For this review, take the finished solid that the model builds, in its own axes (mm). Face numbers are marked on the shaded views. Coordinates: 2 decimals unless noted, no trailing zeros. Write each loop counter-clockwise with the first axis right and the second up, starting at its lowest first coordinate (ties: lowest second). Pieces come first, ordered by that corner, then holes. Notation, with made-up numbers: (34, 74.5) -> (65, 74.5) arc R20 cw to (65, 83.5) -> close; hole circle Ø2 at (20, -35). An arc over 180 degrees is marked (long way). One line per item, written item: value. Start each with the question number.
1) For pin 1 Ø1.5 at (x, z) = (-16, 3.5) entering from +Y; pin 2 Ø5 at (x, y) = (-8, -8.5) entering from -Z; pin 3 Ø3 at (x, y) = (-5.5, -2.5) entering from +Z; pin 4 Ø1.5 at (x, z) = (-18, 2) entering from -Y, all flat-tipped, find the tip position at first contact; note any pin that passes through.
2) Add section C-C (y = 9). State the section outline as (x, z) points.
3) Mouldability with a two-part tool opening along X and no side actions: class the marked faces 1, 2, 3 and 4 as released by +X, released by -X, zero draft, split by the parting line, or undercut.
4) For probe 1 along Y at (x, z) = (-12.5, 4.7); probe 2 along Z at (x, y) = (-5.5, -6); probe 3 along Y at (x, z) = (-5, 0.6) (3 decimals), list the stretches that pass through material, from the lowest coordinate up. Write a range as from..to.
5) Add section A-A (x = -3.75). State the section outline as (y, z) points, and give its area (3 significant figures).
6) Add section B-B (y = 0). State the section outline as (x, z) points, and give its area (3 significant figures).
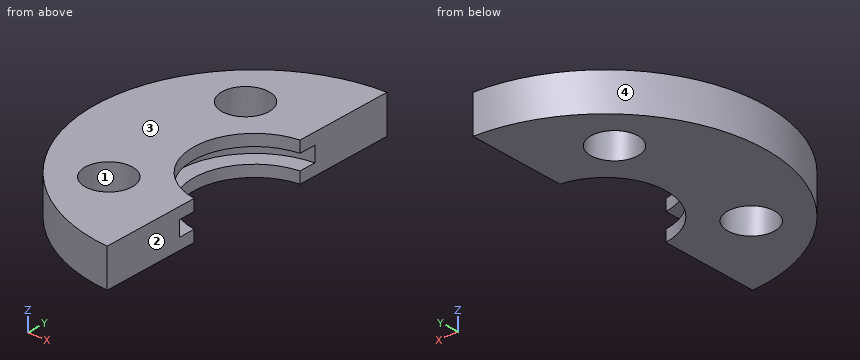
from build123d import *

# Parameters (mm, degrees)
SKETCH_1_R          = 21
SKETCH_1_R_2        = 3.1
SKETCH_1_R_3        = 8
EXTRUDE_1_DEPTH     = 5
CUT_EXTRUDE_1_DEPTH = 10
SKETCH_3_W          = 2
SKETCH_3_H          = 1.455022594
CUT_EXTRUDE_2_DEPTH = 2
SKETCH_4_R          = 10.2
CUT_EXTRUDE_3_DEPTH = 2


with BuildPart() as part:
    # 草图1 → 凸台-拉伸1 (new body)
    with BuildSketch(Plane.XY):
        Circle(SKETCH_1_R)
        with Locations((-10.253048327, 10.253048327)):
            Circle(SKETCH_1_R_2, mode=Mode.SUBTRACT)
        with Locations((10.253048327, 10.253048327)):
            Circle(SKETCH_1_R_2, mode=Mode.SUBTRACT)
        with Locations((-10.253048327, -10.253048327)):
            Circle(SKETCH_1_R_2, mode=Mode.SUBTRACT)
        with Locations((10.253048327, -10.253048327)):
            Circle(SKETCH_1_R_2, mode=Mode.SUBTRACT)
        Circle(SKETCH_1_R_3, mode=Mode.SUBTRACT)
    extrude(amount=EXTRUDE_1_DEPTH)

    # 草图2 → 切除-拉伸1 (cut)
    with BuildSketch(Plane.XY.offset(5)):
        Polygon((-1, 0), (-1, 23.542037427), (27.759132826, 23.542037427), (27.759132826, -27.308763415), (-1, -27.308763415), align=None)
    extrude(amount=-CUT_EXTRUDE_1_DEPTH, mode=Mode.SUBTRACT)

    # 草图3 → 切除-拉伸2 (cut)
    with BuildSketch(Plane(origin=(-1, 0, 0), x_dir=(0, 0, -1), z_dir=(1, 0, 0))):
        with Locations((-2.5, 7.937253933)):
            Rectangle(SKETCH_3_W, SKETCH_3_H)
    extrude(amount=-CUT_EXTRUDE_2_DEPTH, mode=Mode.SUBTRACT)

    # 草图4 → 切除-拉伸3 (cut)
    with BuildSketch(Plane.XY.offset(1.5)):
        Circle(SKETCH_4_R)
    extrude(amount=CUT_EXTRUDE_3_DEPTH, mode=Mode.SUBTRACT)


solid = part.part
Numbers:
1. pin 1: y = 14.44
1. pin 2: z = 0
1. pin 3: through
1. pin 4: y = -11.98
2. outline: (-18.97, 0) -> (-13.09, 0) -> (-13.09, 5) -> (-18.97, 5) -> close; (-7.42, 0) -> (-1, 0) -> (-1, 1.5) -> (-4.8, 1.5) -> (-4.8, 3.5) -> (-1, 3.5) -> (-1, 5) -> (-7.42, 5) -> close
3. face 1: undercut
3. face 2: released by +X
3. face 3: zero draft
3. face 4: released by -X
4. probe 1: -16.87..-12.39, -8.12..8.12, 12.39..16.87
4. probe 2: 0..1.5, 3.5..5
4. probe 3: -20.396..-6.245, 6.245..20.396
5. outline: (-20.66, 0) -> (-7.07, 0) -> (-7.07, 1.5) -> (-9.49, 1.5) -> (-9.49, 3.5) -> (-7.07, 3.5) -> (-7.07, 5) -> (-20.66, 5) -> close; (7.07, 0) -> (20.66, 0) -> (20.66, 5) -> (7.07, 5) -> (7.07, 3.5) -> (9.49, 3.5) -> (9.49, 1.5) -> (7.07, 1.5) -> close
5. area: 126 mm²
6. outline: (-21, 0) -> (-8, 0) -> (-8, 1.5) -> (-10.2, 1.5) -> (-10.2, 3.5) -> (-8, 3.5) -> (-8, 5) -> (-21, 5) -> close
6. area: 60.6 mm²
